from build123d import *

# Parameters (mm, degrees)
F1_DEPTH = 165
F2_W     = 40
F2_H     = 30
F3_DEPTH = 35.001
F4_W     = 40
F4_H     = 30
F5_DEPTH = 12


with BuildPart() as f1:
    # F0 (on Front) → F1 (new body)
    with BuildSketch(Plane.XZ):
        Polygon((0, 51.518065), (0, 31.518065), (300, 31.518065), (300, 66.518065), align=None)
    extrude(amount=F1_DEPTH)

    # F2 (on face) → F3 (cut, through all)
    with BuildSketch(Plane(origin=(0, 0, 31.518065), x_dir=(1, 0, 0), z_dir=(0, 0, -1))):
        with Locations((200, 52.5)):
            Rectangle(F2_W, F2_H)
    extrude(amount=-F3_DEPTH, mode=Mode.SUBTRACT)

    # F4 (on face) → F5 (cut)
    with BuildSketch(Plane(origin=(0, 0, 31.518065), x_dir=(1, 0, 0), z_dir=(0, 0, -1))):
        with BuildLine():
            Line((170, 72.5), (170, 32.5))
            ThreePointArc((170, 32.5), (171.464466, 28.964466), (175, 27.5))
            Line((175, 27.5), (225, 27.5))
            ThreePointArc((225, 27.5), (228.535534, 28.964466), (230, 32.5))
            Line((230, 32.5), (230, 72.5))
            ThreePointArc((230, 72.5), (228.535534, 76.035534), (225, 77.5))
            Line((225, 77.5), (175, 77.5))
            ThreePointArc((175, 77.5), (171.464466, 76.035534), (170, 72.5))
        make_face()
        with Locations((200, 52.5)):
            Rectangle(F4_W, F4_H, mode=Mode.SUBTRACT)
    extrude(amount=-F5_DEPTH, mode=Mode.SUBTRACT)


solid = f1.part
Could you check a few things on this model? Use its own coordinates, in mm. A direction names the side the tool comes from. Give positions to 0.01 mm unless a question says otherwise; leave off trailing zeros. Order: outer loops, then holes, each group sorted by start corner. A loop starts at its lowest first (then second) coordinate and runs counter-clockwise, first axis right, second up.
1. Which directions (+Z, -Z, +X, -X, +Y, -Y) give clear straight access to the entire face, cutting with the end or side of a thin tool? Please do faces 1 (the flat face through (230, -52, 37)), 2 (the flat face through (148, 0, 45)), 3 (the flat face through (180, -52, 52)).
Answers below:
face 1: -Z
face 2: +Z, -Z, +X, -X, +Y
face 3: +Z, -Z
2. I need wall thicknesses on L1, parallel to X at y = -57, z = 46; L2, parallel to Y at x = 190, z = 41.5; L3, parallel to X at y = -72.5, z = 40.5. Which ranges of each line are inside material? Lowest first, please.
Answers below:
L1: x = 0 to 180, 220 to 300
L2: y = -165 to -77.5, -27.5 to 0
L3: x = 0 to 170, 230 to 300
3. For pin 1 (4 mm diameter, centred on x = 87, y = -129.5, fed in from +Z); pin 2 (1 mm diameter, centred on x = 225, y = -58.5, fed in from +Z); pin 3 (6 mm diameter, centred on y = -44.5, z = 36, fed in from -X); pin 4 (10 mm diameter, centred on x = 215, y = -69.5, fed in from +Z), each with a flat end and sliding along its axis, tell me the tip position at first contact or that it passes through.
Answers below:
pin 1: stops at z = 55.97
pin 2: stops at z = 62.79
pin 3: stops at x = 0
pin 4: stops at z = 62.52
4. Suppose I cut it at B-B (y = -47.5). Write out the boundary of the cut face in (x, z), plus the area to 3 significant figures.
Answers below:
outline: (0, 31.52) - (170, 31.52) - (170, 43.52) - (180, 43.52) - (180, 60.52) - (0, 51.52) - close; (220, 43.52) - (230, 43.52) - (230, 31.52) - (300, 31.52) - (300, 66.52) - (220, 62.52) - close
area: 6,810 mm2
5. Suppose I cut it at D-D (y = -139.5). Write out the boundary of the cut face in (x, z).
Answers below:
outline: (0, 31.52) - (300, 31.52) - (300, 66.52) - (0, 51.52) - close
6. Suppose I cut it at C-C (x = 191.5). Write out the boundary of the cut face in (y, z).
Answers below:
outline: (-165, 31.52) - (-77.5, 31.52) - (-77.5, 43.52) - (-67.5, 43.52) - (-67.5, 61.09) - (-165, 61.09) - close; (-37.5, 43.52) - (-27.5, 43.52) - (-27.5, 31.52) - (0, 31.52) - (0, 61.09) - (-37.5, 61.09) - close
7. Thinking about a two-plate mould opening in Y: for faces 4 (the flat face through (220, -52, 53)), 5 (the flat face through (0, -81, 42)), 6 (the flat face through (148, -165, 45)), 7 (the flat face through (200, -70, 43.518)), which applies, +Y half, -Y half, draft (parallel to the pull), parting line (faces both ways), or undercut?
Answers below:
face 4: undercut
face 5: draft
face 6: -Y half
face 7: undercut
8. Suppose I cut it at A-A (z = 35.5). Write out the boundary of the cut face in (x, y), plus the area to 3 significant figures.
Answers below:
outline: (0, -165) - (300, -165) - (300, 0) - (0, 0) - close; hole (170, -72.5) arc R5 ccw to (175, -77.5) - (225, -77.5) arc R5 ccw to (230, -72.5) - (230, -32.5) arc R5 ccw to (225, -27.5) - (175, -27.5) arc R5 ccw to (170, -32.5) - close
area: 46,500 mm2
